Verification items for the finished model (mm, model axes). Face numbers are marked on the shaded views. A direction names the side the tool comes from. Give positions to 0.01 mm unless a question says otherwise; leave off trailing zeros. Order: outer loops, then holes, each group sorted by start corner. A loop starts at its lowest first (then second) coordinate and runs counter-clockwise, first axis right, second up. Notation, with made-up numbers: (-23.75, 69.5) - (17.25, 69.5) arc R5 ccw to (17.25, 74.5) - close; hole circle Ø6 at (23.25, 37.5). An arc over 180 degrees is marked (long way). Answer as a JSON object with one key per item and string values.
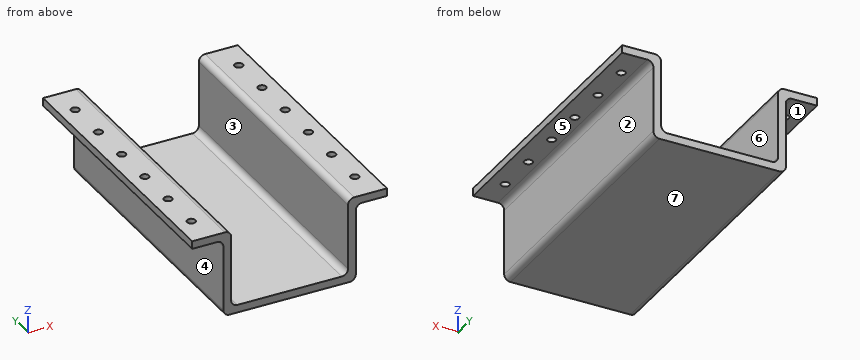
```python
from build123d import *

# Parameters (mm, degrees)
F1_DEPTH = 228.6
F3_R     = 5.08
F6_D     = 6.7564
F7_D     = 6.7564


with BuildPart() as f1:
    # F0 (on Front) → F1 (new body)
    with BuildSketch(Plane.XZ):
        Polygon((-53.975, 63.5), (-53.975, 0), (53.975, 0), (53.975, 63.5), (79.375, 63.5), (79.375, 69.85), (47.625, 69.85), (47.625, 6.35), (-47.625, 6.35), (-47.625, 69.85), (-79.375, 69.85), (-79.375, 63.5), align=None)
    extrude(amount=-F1_DEPTH)

    # F3
    f3_edges = [f1.edges().sort_by_distance(p)[0] for p in [
        (-47.625, 114.3, 69.85),
        (-47.625, 114.3, 6.35),
        (53.975, 114.3, 0),
        (47.625, 114.3, 6.35),
        (-53.975, 114.3, 0),
        (-53.975, 114.3, 63.5),
        (53.975, 114.3, 63.5),
        (47.625, 114.3, 69.85),
    ]]
    fillet(f3_edges, radius=F3_R)

    # F6 (through all)
    with Locations(Plane.XY.offset(69.85)):
        with Locations((-66.675, 203.2), (-66.675, 167.64), (-66.675, 132.08), (-66.675, 96.52), (-66.675, 60.96), (-66.675, 25.4)):
            Hole(F6_D / 2)

    # F7 (through all)
    with Locations(Plane.XY.offset(69.85)):
        with Locations((66.675, 203.2), (66.675, 167.64), (66.675, 132.08), (66.675, 96.52), (66.675, 60.96), (66.675, 25.4)):
            Hole(F7_D / 2)


solid = f1.part
```
(1) Access from +Z, -Z, +X, -X, +Y, -Y to the whole of each face (thin tool, end or side, straight path). Record for the marked faces 5, 6 and 7.
Computed values:
{"face 5": "-Z, +X, +Y, -Y", "face 6": "+Z, +Y, -Y", "face 7": "-Z, +X, -X, +Y, -Y"}
(2) Gauge pin test, flat ends, axial feed: pin 1 Ø4 at (x, y) = (66.675, 25.4) entering from +Z (3 decimals); pin 2 Ø3 at (x, y) = (35.5, 55.5) entering from +Z; pin 3 Ø9 at (x, y) = (-66.675, 60.96) entering from -Z; pin 4 Ø9 at (x, y) = (66.675, 60.96) entering from +Z. Record the tip position at first contact, or that the pin passes through.
Computed values:
{"pin 1": "passes through", "pin 2": "stops at z = 6.35", "pin 3": "stops at z = 63.5", "pin 4": "stops at z = 69.85"}
(3) Material ranges on line 1 along X through (y, z) = (183.5, 57.5) (3 decimals); line 2 along X through (y, z) = (167, 67) (3 decimals); line 3 along Z through (x, y) = (-25, 139), recorded low to high. Write a range as [from, to].
Computed values:
{"line 1": "x = [-53.975, -47.625], [47.625, 53.975]", "line 2": "x = [-79.375, -69.992], [-63.358, -48.141], [48.141, 63.358], [69.992, 79.375]", "line 3": "z = [0, 6.35]"}
(4) Release check for a two-part mould opening along X. For the marked faces 1, 2, 3 and 4 record: pulls with the +X half, pulls with the -X half, needs draft (parallel to the pull), parting line crosses it, or undercut.
Computed values:
{"face 1": "needs draft", "face 2": "pulls with the +X half", "face 3": "undercut", "face 4": "pulls with the -X half"}
(5) Section check D-D (y = 46). Record the cut outline in (x, z) (3 decimals), then the cut area to 3 significant figures.
Computed values:
{"outline": "(-79.375, 63.5) - (-59.055, 63.5) arc R5.08 cw to (-53.975, 58.42) - (-53.975, 5.08) arc R5.08 ccw to (-48.895, 0) - (48.895, 0) arc R5.08 ccw to (53.975, 5.08) - (53.975, 58.42) arc R5.08 cw to (59.055, 63.5) - (79.375, 63.5) - (79.375, 69.85) - (52.705, 69.85) arc R5.08 ccw to (47.625, 64.77) - (47.625, 11.43) arc R5.08 cw to (42.545, 6.35) - (-42.545, 6.35) arc R5.08 cw to (-47.625, 11.43) - (-47.625, 64.77) arc R5.08 ccw to (-52.705, 69.85) - (-79.375, 69.85) - close", "area": "1,810 mm²"}
(6) Section check A-A (z = 23.5). Record the cut outline in (x, y) (3 decimals), then the cut area to 3 significant figures.
Computed values:
{"outline": "(-53.975, 0) - (-47.625, 0) - (-47.625, 228.6) - (-53.975, 228.6) - close; (47.625, 0) - (53.975, 0) - (53.975, 228.6) - (47.625, 228.6) - close", "area": "2,900 mm²"}
(7) Section check B-B (y = 96.52). Record the cut outline in (x, z) (3 decimals), then the cut area to 3 significant figures.
Computed values:
{"outline": "(-79.375, 63.5) - (-70.053, 63.5) - (-70.053, 69.85) - (-79.375, 69.85) - close; (-63.297, 63.5) - (-59.055, 63.5) arc R5.08 cw to (-53.975, 58.42) - (-53.975, 5.08) arc R5.08 ccw to (-48.895, 0) - (48.895, 0) arc R5.08 ccw to (53.975, 5.08) - (53.975, 58.42) arc R5.08 cw to (59.055, 63.5) - (63.297, 63.5) - (63.297, 69.85) - (52.705, 69.85) arc R5.08 ccw to (47.625, 64.77) - (47.625, 11.43) arc R5.08 cw to (42.545, 6.35) - (-42.545, 6.35) arc R5.08 cw to (-47.625, 11.43) - (-47.625, 64.77) arc R5.08 ccw to (-52.705, 69.85) - (-63.297, 69.85) - close; (70.053, 63.5) - (79.375, 63.5) - (79.375, 69.85) - (70.053, 69.85) - close", "area": "1,730 mm²"}
(8) Section check C-C (x = -25). Record the cut outline in (y, z).
Computed values:
{"outline": "(0, 0) - (228.6, 0) - (228.6, 6.35) - (0, 6.35) - close"}
